```python
from build123d import *

# Parameters (mm, degrees)
F0_W      = 6.75
F0_H      = 32
F0_W_2    = 11.5
F0_R      = 3.35
F1_DEPTH  = 12
F2_DEPTH  = 20
F3_SIZE   = 5
F4_SIZE   = 5
F6_D      = 5.5
F8_DEPTH  = 4.1
F10_SIZE  = 0.5
F9_W      = 12.25
F9_H      = 0.5
F9_W_2    = 0.5
F9_H_2    = 15.75
F11_DEPTH = 0.5


# Not quite as in the source:
# - a pattern or mirror of a feature is missing from the dataset's text; its kind, count and spacing are read off the source's solid


with BuildPart() as f1:
    # F0 (on Top) → F1 (new body)
    with BuildSketch(Plane.XY):
        with Locations((9.125, 0)):
            Rectangle(F0_W, F0_H)
        Rectangle(F0_W_2, F0_H)
        Circle(F0_R, mode=Mode.SUBTRACT)
        with Locations((-9.125, 0)):
            Rectangle(F0_W, F0_H)
    extrude(amount=F1_DEPTH)

    # F0 (on Top) → F2 (join)
    with BuildSketch(Plane.XY):
        with Locations((9.125, 0)):
            Rectangle(F0_W, F0_H)
        with Locations((-9.125, 0)):
            Rectangle(F0_W, F0_H)
    extrude(amount=-F2_DEPTH)

    # F3
    f3_edges = [f1.edges().sort_by_distance(p)[0] for p in [
        (-9.125, -16, -20),
        (9.125, -16, -20),
        (9.125, 16, -20),
        (-9.125, 16, -20),
    ]]
    chamfer(f3_edges, length=F3_SIZE)

    # F4
    f4_edges = [f1.edges().sort_by_distance(p)[0] for p in [
        (0, -16, 12),
        (0, 16, 12),
    ]]
    chamfer(f4_edges, length=F4_SIZE)

    # F6 (through all)
    with Locations(Plane(origin=(-12.5, 0, 0), x_dir=(0, -1, 0), z_dir=(-1, 0, 0))):
        with Locations((0, -10)):
            Hole(F6_D / 2)

    # F7 (on face) → F8 (cut)
    with BuildSketch(Plane(origin=(5.75, 0, 0), x_dir=(0, -1, 0), z_dir=(-1, 0, 0))):
        Polygon((4.1, -12.3671361037), (4.1, -7.6328638963), (0, -5.2657277926), (-4.1, -7.6328638963), (-4.1, -12.3671361037), (0, -14.7342722074), align=None)
    f8 = extrude(amount=-F8_DEPTH, mode=Mode.SUBTRACT)

    # F8_copies: F8 across plane
    add(f8.mirror(Plane(origin=(0, 0, 0), x_dir=(0, 0, -1), z_dir=(-1, 0, 0))), mode=Mode.SUBTRACT)

    # F10
    f10_edges = [f1.edges().sort_by_distance(p)[0] for p in [
        (12.5, 0, 12),
        (12.5, -13.5, 9.5),
        (12.5, -16, -4),
        (12.5, -13.5, -17.5),
        (12.5, 0, -20),
        (12.5, 13.5, -17.5),
        (12.5, 16, -4),
        (12.5, 13.5, 9.5),
        (-12.5, -16, -4),
        (-12.5, -13.5, 9.5),
        (-12.5, -13.5, -17.5),
        (-12.5, 0, 12),
        (-12.5, 0, -20),
        (-12.5, 13.5, 9.5),
        (-12.5, 13.5, -17.5),
        (-12.5, 16, -4),
        (-12.5, 2.75, -10),
        (0, 16, 0),
        (0, -16, 0),
        (5.75, -16, -7.5),
        (5.75, -13.5, -17.5),
        (5.75, 0, -20),
        (5.75, 13.5, -17.5),
        (5.75, 16, -7.5),
        (-5.75, 16, -7.5),
        (-5.75, 13.5, -17.5),
        (-5.75, 0, -20),
        (-5.75, -13.5, -17.5),
        (-5.75, -16, -7.5),
        (-3.35, 0, 12),
        (-3.35, 0, 0),
        (12.5, 2.75, -10),
    ]]
    chamfer(f10_edges, length=F10_SIZE)

    # F9 (on face) → F11 (cut)
    with BuildSketch(Plane.XY.offset(12)):
        with Locations((-6.375, 0)):
            Rectangle(F9_W, F9_H)
        Rectangle(F9_W_2, F9_H)
        with Locations((0, -8.125)):
            Rectangle(F9_W_2, F9_H_2)
        with Locations((6.375, 0)):
            Rectangle(F9_W, F9_H)
        with Locations((0, 8.125)):
            Rectangle(F9_W_2, F9_H_2)
    extrude(amount=-F11_DEPTH, mode=Mode.SUBTRACT)


solid = f1.part
```
Input: part model. Units: mm. Frame: model coordinates. A direction names the side the tool comes from. Round coordinates to 2 decimals unless told otherwise and drop trailing zeros. Loops run counter-clockwise (first coordinate to the right, second up) from the corner with the lowest first, then second, coordinate; pieces in that order, holes last. Notation, with made-up numbers: (34, 24.25) -> (84, 24.25) arc R21 ccw to (84, 49.25) -> close; hole circle Ø2 at (-6.5, 36.5). An arc over 180 degrees is marked (long way). Use one line per item in the form item = value. Start each with the question number.
Item 1: Section query A-A on z = -2. Return the cut outline in (x, y), then the cut area to 3 significant figures.
Item 2: Contact query for flat-ended pins moving along their axis: pin 1 Ø0.6 at (x, z) = (8.5, 11.5) entering from +Y; pin 2 Ø6 at (x, y) = (-7.5, -13) entering from +Z; pin 3 Ø9 at (x, y) = (1, -3.5) entering from -Z; pin 4 Ø0.6 at (x, z) = (7, 11.5) entering from -Y. Output: stop coordinate, or through.
Item 3: Mould query, pull axis Z, two halves, no side actions, for faces 5 (the face through (9, -14, -17)), 6 (the face through (-7.77, 2.02, -6.43)), 7 (the face through (6, -6, 12)). Classes: pulls with the +Z half, pulls with the -Z half, needs draft (parallel to the pull), parting line crosses it, or undercut.
Item 4: Section query B-B on y = 5.5. Return the cut outline in (x, z).
Item 5: Section query C-C on x = 5. Return the cut outline in (y, z), then the cut area to 4 significant figures.
Item 6: Section query D-D on z = 9.5. Return the cut outline in (x, y), then the cut area to 3 significant figures.
Item 7: Material intervals for L1, parallel to Z at x = -10.3, y = 0; L2, parallel to Y at x = 0, z = 3; L3, parallel to X at y = -11, z = -1, sorted ascending. Write a range as from..to.
Item 8: Set-up query: faces 1 (the face through (-9, -14, -17)), 2 (the face through (6, 13.29, -17.36)), 3 (the face through (7.77, -2.02, -13.57)), 4 (the face through (2.489, 2.44, 11.635)). Return all of +Z, -Z, +X, -X, +Y, -Y with unobstructed straight access to the full face (end or side cutting, diameter ignored); none if empty.
Ans:
q1.outline = (-12.5, -15.5) -> (-12, -16) -> (-6.25, -16) -> (-5.75, -15.5) -> (-5.75, 15.5) -> (-6.25, 16) -> (-12, 16) -> (-12.5, 15.5) -> close; (5.75, -15.5) -> (6.25, -16) -> (12, -16) -> (12.5, -15.5) -> (12.5, 15.5) -> (12, 16) -> (6.25, 16) -> (5.75, 15.5) -> close
q1.area = 431 mm^2
q2.pin_1 = 11.8
q2.pin_2 = 12
q2.pin_3 = 0
q2.pin_4 = -11.8
q3.face_5 = pulls with the -Z half
q3.face_6 = undercut
q3.face_7 = pulls with the +Z half
q4.outline = (-12.5, -19.5) -> (-12, -20) -> (-6.25, -20) -> (-5.75, -19.5) -> (-5.75, 0) -> (5.75, 0) -> (5.75, -19.5) -> (6.25, -20) -> (12, -20) -> (12.5, -19.5) -> (12.5, 11.5) -> (12, 12) -> (0.25, 12) -> (0.25, 11.5) -> (-0.25, 11.5) -> (-0.25, 12) -> (-12, 12) -> (-12.5, 11.5) -> close
q5.outline = (-16, 0.5) -> (-15.5, 0) -> (15.5, 0) -> (16, 0.5) -> (16, 7) -> (11, 12) -> (0.25, 12) -> (0.25, 11.5) -> (-0.25, 11.5) -> (-0.25, 12) -> (-11, 12) -> (-16, 7) -> close
q5.area = 358.5 mm^2
q6.outline = (-12.5, -12.79) -> (-12, -13.5) -> (12, -13.5) -> (12.5, -12.79) -> (12.5, 12.79) -> (12, 13.5) -> (-12, 13.5) -> (-12.5, 12.79) -> close; hole circle Ø6.7 at (0, 0)
q6.area = 639 mm^2
q7.L1 = -20..-12.75, -7.25..11.5
q7.L2 = -16..-3.35, 3.35..16
q7.L3 = -12.5..-5.75, 5.75..12.5
q8.face_1 = -Z, +X, -X, -Y
q8.face_2 = -Z, +Y
q8.face_3 = none
q8.face_4 = +Z
